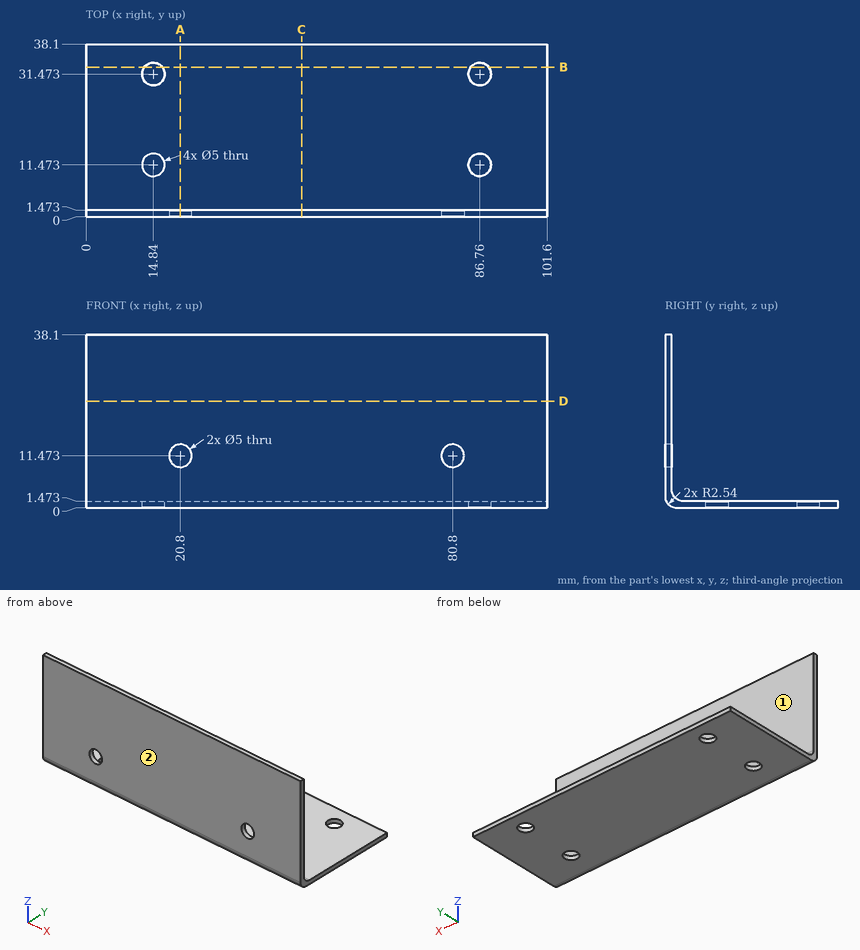
Could you check a few things on this drawing? It's one solid part, dimensions in mm from its lowest x, y, z. A direction names the side the tool comes from. Round coordinates to 2 decimals unless told otherwise and drop trailing zeros. Loops run counter-clockwise (first coordinate to the right, second up) from the corner with the lowest first, then second, coordinate; pieces in that order, holes last.
Q1. Please list where this line runs through material, in increasing order: L1, parallel to Z at x = 19.5, y = 19.
Q2. I want a section at D-D (z = 23.5). Write out the boundary of the cut face in (x, y).
Q3. I want a section at B-B (y = 33). Write out the boundary of the cut face in (x, z).
Q4. On a 3-axis mill with a long thin cutter (end or side, diameter ignored), from which of +Z, -Z, +X, -X, +Y, -Y can I reach the whole of each face in a straight line? I mean the marked faces 1 and 2. Say none if no direction works.
Q5. I want a section at C-C (x = 47.5). Write out the boundary of the cut face in (y, z).
Q6. For P1, Ø3, axis at x = 14.84, y = 31.47, coming from the +Z side, with a flat end and sliding along its axis, tell me the tip position at first contact or that it passes through.
Q7. I want a section at A-A (x = 20.8). Write out the boundary of the cut face in (y, z).
Answer below:
1. L1: z = 0 to 1.47
2. outline: (0, 0) - (101.6, 0) - (101.6, 1.47) - (0, 1.47) - close
3. outline: (0, 0) - (12.86, 0) - (12.86, 1.47) - (0, 1.47) - close; (16.82, 0) - (84.78, 0) - (84.78, 1.47) - (16.82, 1.47) - close; (88.74, 0) - (101.6, 0) - (101.6, 1.47) - (88.74, 1.47) - close
4. face 1: +Z, +X, -X, +Y
4. face 2: +Z, -Z, +X, -X, -Y
5. outline: (0, 2.54) arc R2.54 ccw to (2.54, 0) - (38.1, 0) - (38.1, 1.47) - (4.01, 1.47) arc R2.54 cw to (1.47, 4.01) - (1.47, 38.1) - (0, 38.1) - close
6. P1: passes through
7. outline: (0, 2.54) arc R2.54 ccw to (2.54, 0) - (38.1, 0) - (38.1, 1.47) - (4.01, 1.47) arc R2.54 cw to (1.47, 4.01) - (1.47, 8.97) - (0, 8.97) - close; (0, 13.97) - (1.47, 13.97) - (1.47, 38.1) - (0, 38.1) - close
